```python
from build123d import *

# Parameters (mm, degrees)
SKETCH1_R                = 8
SKETCH1_R_2              = 5
BOSS_EXTRUDE1_DEPTH      = 8
WRAP2_SECTION_W          = 4
WRAP2_SECTION_H          = 5
WRAP2_ANGLE              = 21.485917317
WRAP2_SECTOR_2_SECTION_W = 4
WRAP2_SECTOR_2_SECTION_H = 5
WRAP2_SECTOR_2_ANGLE     = 21.485917317


with BuildPart() as part:
    # Sketch1 → Boss-Extrude1 (new body)
    with BuildSketch(Plane.XY):
        Circle(SKETCH1_R)
        Circle(SKETCH1_R_2, mode=Mode.SUBTRACT)
    extrude(amount=BOSS_EXTRUDE1_DEPTH)

    # Wrap2 section (on wrap section) → Wrap2 (revolve, cut)
    with BuildSketch(Plane(origin=(0, 0, 0), x_dir=(-0.9691091288804563, -0.24663230996883403, 0), z_dir=(0.24663230996883403, -0.9691091288804563, 0))):
        with Locations((6, -5.5)):
            Rectangle(WRAP2_SECTION_W, WRAP2_SECTION_H)
    revolve(axis=Axis((0, 0, 0), (0, 0, -1)), revolution_arc=WRAP2_ANGLE, mode=Mode.SUBTRACT)

    # Wrap2 sector 2 section (on wrap section) → Wrap2 sector 2 (revolve, cut)
    with BuildSketch(Plane(origin=(0, 0, 0), x_dir=(0.9687151001182653, 0.24817545165237268, 0), z_dir=(-0.24817545165237268, 0.9687151001182653, 0))):
        with Locations((6, -5.5)):
            Rectangle(WRAP2_SECTOR_2_SECTION_W, WRAP2_SECTOR_2_SECTION_H)
    revolve(axis=Axis((0, 0, 0), (0, 0, -1)), revolution_arc=WRAP2_SECTOR_2_ANGLE, mode=Mode.SUBTRACT)


solid = part.part
```
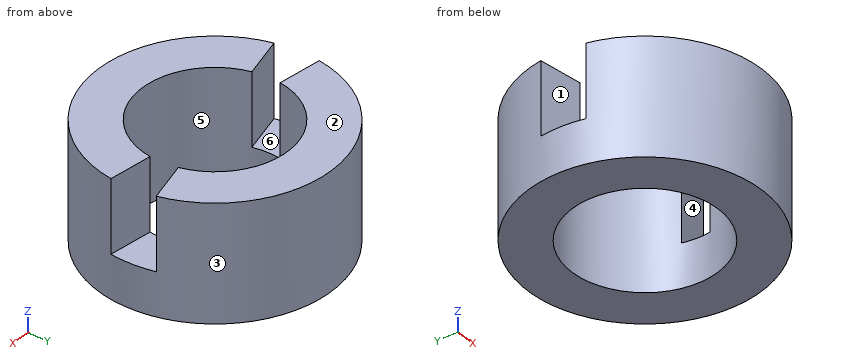
Geometry check sheet. Reference: the model listing, model coordinates, mm. Face numbers are marked on the shaded views. A direction names the side the tool comes from. Give positions to 0.01 mm unless a question says otherwise; leave off trailing zeros. Loops run counter-clockwise (first coordinate to the right, second up) from the corner with the lowest first, then second, coordinate; pieces in that order, holes last. Notation, with made-up numbers: M 66,26 L 124,26 A15 cw 124,41 Z; hole C 39,80.25 d11. An arc over 180 degrees is marked long. Write item = value, one per line. Start each with the question number.
1. Section check D-D, the plane x = 6. Enter the section's corners in (y, z), plus the area to 3 significant figures.
2. Section check A-A, the plane y = 0. Enter the section's corners in (x, z), plus the area to 3 significant figures.
3. Section check B-B, the plane z = 4.5. Enter the section's corners in (x, y).
4. Tool access check on the marked faces 4, 5 and 6. Record the directions out of +Z, -Z, +X, -X, +Y, -Y that give a thin tool (end or side, any length) a straight path to the whole face; none if there is none.
5. Thickness scan on probe 1 along Y at (x, z) = (0, 5.25); probe 2 along Y at (x, z) = (-2.5, 7.75). Record the ranges inside material, lowest first.
6. Go/stop test with flat-tipped pins: P1, Ø1.5, axis at y = 2, z = 1, coming from the +X side; P2, Ø1, axis at x = 3, z = 4, coming from the +Y side; P3, Ø1.5, axis at x = 1.5, z = 6, coming from the +Y side. Record where each tip stops, or that it passes through.
7. Section check C-C, the plane z = 1.75. Enter the section's corners in (x, y).
8. Draft check along Y on the marked faces 1, 2 and 3. Enter one of: +Y half, -Y half, draft (parallel to the pull), parting line (faces both ways), or undercut.
Values follow:
q1.outline = M -5.29,0 L 5.29,0 L 5.29,8 L 1.54,8 L 1.54,3 L -0.75,3 L -0.75,8 L -5.29,8 Z
q1.area = 73.2 mm^2
q2.outline = M -8,0 L -5,0 L -5,3 L -8,3 Z; M 5,0 L 8,0 L 8,3 L 5,3 Z
q2.area = 18.0 mm^2
q3.outline = M -7.94,1 L -4.96,0.63 A5 cw 4.84,1.24 L 7.75,1.99 A8 ccw Z; M -7.75,-1.97 A8 ccw 7.94,-0.99 L 4.96,-0.62 A5 cw -4.85,-1.23 Z
q4.face_4 = +Z, +X
q4.face_5 = +Z, -Z
q4.face_6 = +Z, -X
q5.probe_1 = -8 to -5, 5 to 8
q5.probe_2 = -7.6 to -4.33, 4.33 to 7.6
q6.P1 = 7.9
q6.P2 = 7.6
q6.P3 = 7.96
q7.outline = C 0,0 d16; hole C 0,0 d10
q8.face_1 = undercut
q8.face_2 = draft
q8.face_3 = parting line
